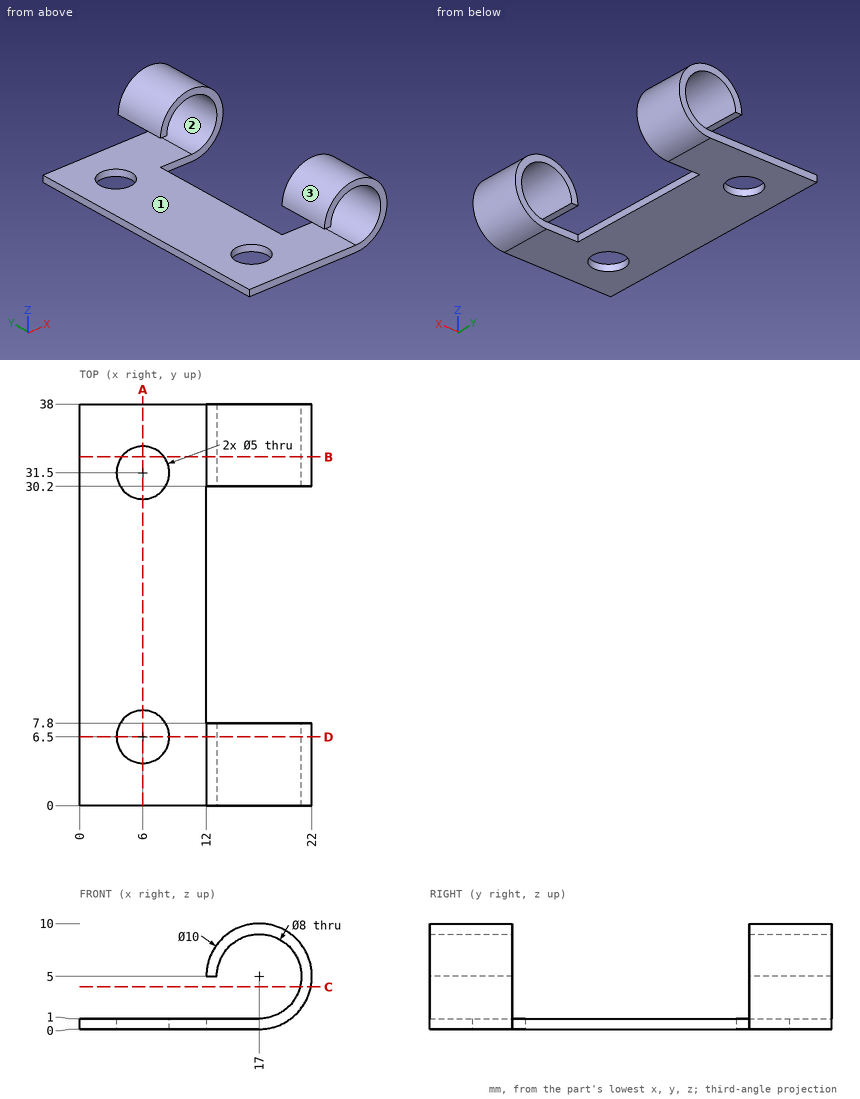
Answer from the drawing. Dimensions are ordinates in mm from the lowest x, y and z of the part. Round coordinates to 2 decimals unless told otherwise and drop trailing zeros. Order: outer loops, then holes, each group sorted by start corner. A loop starts at its lowest first (then second) coordinate and runs counter-clockwise, first axis right, second up.
1) Flat-ended cylindrical pins translate along their axes: pin 1 (0.8 mm diameter, centred on x = 12.5, y = 4, fed in from -Z); pin 2 (2 mm diameter, centred on x = 18, z = 7, fed in from -Y); pin 3 (0.8 mm diameter, centred on y = 15, z = 0.5, fed in from +X); pin 4 (2 mm diameter, centred on y = 6, z = 3, fed in from +X). Find the tip coordinate at first contact, or state that the pin passes through.
2) The part is cut by section B-B on y = 33. Write down the section's boundary in (x, z).
3) The part is cut by section A-A on x = 6. Write down the section's boundary in (y, z).
4) The mould has two halves that part along X. Classify the marked faces 1, 2 and 3: released by +X, released by -X, zero draft, split by the parting line, or undercut.
5) Straight lines are drawn through the part: L1, parallel to Z at x = 17, y = 35.25; L2, parallel to Y at x = 20.5, z = 7.5; L3, parallel to Y at x = 6, z = 0.4. For each, find the intervals that lie inside material, in ascending order.
6) The part is cut by section D-D on y = 6.5. Write down the section's boundary in (x, z).
7) The part is cut by section C-C on z = 4. Write down the section's boundary in (x, y), plus the area to 3 significant figures.
Resolved:
1. pin 1: stops at z = 0
1. pin 2: passes through
1. pin 3: stops at x = 12
1. pin 4: stops at x = 21.9
2. outline: (0, 0) - (4, 0) - (4, 1) - (0, 1) - close; (8, 0) - (17, 0) arc R5 ccw (long way) to (12, 5) - (13, 5) arc R4 cw (long way) to (17, 1) - (8, 1) - close
3. outline: (0, 0) - (4, 0) - (4, 1) - (0, 1) - close; (9, 0) - (29, 0) - (29, 1) - (9, 1) - close; (34, 0) - (38, 0) - (38, 1) - (34, 1) - close
4. face 1: zero draft
4. face 2: undercut
4. face 3: split by the parting line
5. L1: z = 0 to 1, 9 to 10
5. L2: y = 0 to 7.8, 30.2 to 38
5. L3: y = 0 to 4, 9 to 29, 34 to 38
6. outline: (0, 0) - (3.5, 0) - (3.5, 1) - (0, 1) - close; (8.5, 0) - (17, 0) arc R5 ccw (long way) to (12, 5) - (13, 5) arc R4 cw (long way) to (17, 1) - (8.5, 1) - close
7. outline: (20.87, 0) - (21.9, 0) - (21.9, 7.8) - (20.87, 7.8) - close; (20.87, 30.2) - (21.9, 30.2) - (21.9, 38) - (20.87, 38) - close
7. area: 16.0 mm2
